```python
from build123d import *

# Parameters (mm, degrees)
CROQUIS1_W              = 365
CROQUIS1_H              = 80
SALIENTE_EXTRUIR1_DEPTH = 50
REDONDEO1_R             = 20
REDONDEO2_R             = 20
REDONDEO3_R             = 20
REDONDEO4_R             = 20
CROQUIS2_W              = 25
CROQUIS2_H              = 25
SALIENTE_EXTRUIR2_DEPTH = 27
CROQUIS3_W              = 19
CROQUIS3_H              = 19
CORTAR_EXTRUIR1_DEPTH   = 23


with BuildPart() as part:
    # Croquis1 → Saliente-Extruir1 (new body)
    with BuildSketch(Plane(origin=(0, 0, 0), x_dir=(1, 0, 0), z_dir=(0, 1, 0))):
        with Locations((-182.5, 40)):
            Rectangle(CROQUIS1_W, CROQUIS1_H)
    extrude(amount=SALIENTE_EXTRUIR1_DEPTH)

    # Redondeo1
    redondeo1_edges = [part.edges().sort_by_distance(p)[0] for p in [
        (-182.5, 50, -80),
    ]]
    fillet(redondeo1_edges, radius=REDONDEO1_R)

    # Redondeo2
    redondeo2_edges = [part.edges().sort_by_distance(p)[0] for p in [
        (-182.5, 50, 0),
    ]]
    fillet(redondeo2_edges, radius=REDONDEO2_R)

    # Redondeo3
    redondeo3_edges = [part.edges().sort_by_distance(p)[0] for p in [
        (0, 15, -80),
        (0, 44.142135624, -74.142135624),
        (0, 15, 0),
        (0, 50, -40),
        (0, 44.142135624, -5.857864376),
    ]]
    fillet(redondeo3_edges, radius=REDONDEO3_R)

    # Redondeo4
    redondeo4_edges = [part.edges().sort_by_distance(p)[0] for p in [
        (-365, 15, -80),
        (-365, 44.142135624, -74.142135624),
        (-365, 15, 0),
        (-365, 50, -40),
        (-365, 44.142135624, -5.857864376),
    ]]
    fillet(redondeo4_edges, radius=REDONDEO4_R)

    # Croquis2 → Saliente-Extruir2 (add)
    with BuildSketch(Plane.XZ):
        with Locations((-53.967193185, -38.316617584)):
            Rectangle(CROQUIS2_W, CROQUIS2_H)
    extrude(amount=SALIENTE_EXTRUIR2_DEPTH)

    # Croquis3 → Cortar-Extruir1 (cut)
    with BuildSketch(Plane.XZ.offset(27)):
        with Locations((-54, -38)):
            Rectangle(CROQUIS3_W, CROQUIS3_H)
    extrude(amount=-CORTAR_EXTRUIR1_DEPTH, mode=Mode.SUBTRACT)


solid = part.part
```
Design review of the part built by this model. Coordinates are the model's own, in mm. A direction names the side the tool comes from. Round coordinates to 2 decimals unless told otherwise and drop trailing zeros. Order: outer loops, then holes, each group sorted by start corner. A loop starts at its lowest first (then second) coordinate and runs counter-clockwise, first axis right, second up. Notation, with made-up numbers: (81.25, -21) - (124.25, -21) arc R24 cw to (124.25, 10) - close; hole circle Ø4 at (69, 62.25). An arc over 180 degrees is marked (long way). Return JSON: item names as keys, results as strings.
Q1. Machinability: for faces 1 (the flat face through (-66.467, -13, -38)), 2 (the flat face through (-54, -13, -50.817)), 3 (the flat face through (-54, -16, -47.5)), which of the approach directions +Z, -Z, +X, -X, +Y, -Y give a long, thin tool a straight path to every point of the face, cutting with its end or side? Answer none if there is none.
Computed values:
{"face 1": "+Z, -Z, -X, -Y", "face 2": "-Z, +X, -X, -Y", "face 3": "-Y"}
Q2. Wall thickness on L1, parallel to X at y = -21, z = -45; L2, parallel to Y at x = -161.5, z = -25.5; L3, parallel to X at y = 31, z = -21.5: over which ranges is each line inside the solid? List them lowest first. Write a range as [from, to].
Computed values:
{"L1": "x = [-66.47, -63.5], [-44.5, -41.47]", "L2": "y = [0, 50]", "L3": "x = [-364.97, -0.03]"}
Q3. Consider section C-C on z = -41. Write out the cut boundary in (x, y), plus the area to 3 significant figures.
Computed values:
{"outline": "(-365, 0) - (-66.47, 0) - (-66.47, -27) - (-63.5, -27) - (-63.5, -4) - (-44.5, -4) - (-44.5, -27) - (-41.47, -27) - (-41.47, 0) - (0, 0) - (0, 30) arc R20 ccw to (-20, 50) - (-345, 50) arc R20 ccw to (-365, 30) - close", "area": "18,300 mm2"}
Q4. Consider section B-B on x = -250.5. Write out the cut boundary in (y, z), plus the area to 3 significant figures.
Computed values:
{"outline": "(0, -80) - (30, -80) arc R20 ccw to (50, -60) - (50, -20) arc R20 ccw to (30, 0) - (0, 0) - close", "area": "3,830 mm2"}
Q5. Consider section A-A on y = -21.5. Write out the cut boundary in (x, z), plus the area to 3 significant figures.
Computed values:
{"outline": "(-66.47, -50.82) - (-41.47, -50.82) - (-41.47, -25.82) - (-66.47, -25.82) - close; hole (-63.5, -47.5) - (-44.5, -47.5) - (-44.5, -28.5) - (-63.5, -28.5) - close", "area": "264 mm2"}
Q6. Consider section D-D on y = 39.5. Write out the cut boundary in (x, z), plus the area to 3 significant figures.
Computed values:
{"outline": "(-362.6, -60) arc R17.6 ccw to (-345, -77.6) - (-20, -77.6) arc R17.6 ccw to (-2.4, -60) - (-2.4, -20) arc R17.6 ccw to (-20, -2.4) - (-345, -2.4) arc R17.6 ccw to (-362.6, -20) - close", "area": "26,800 mm2"}
Q7. For pin 1 Ø15 at (y, z) = (-13, -35) entering from -X; pin 2 Ø5.5 at (x, y) = (-54, -16.5) entering from +Z; pin 3 Ø12.5 at (x, y) = (-57.5, -13.5) entering from -Z, all flat-tipped, find the tip position at first contact; note any pin that passes through.
Computed values:
{"pin 1": "stops at x = -66.47", "pin 2": "stops at z = -25.82", "pin 3": "stops at z = -50.82"}
Q8. The part is to be moulded in two halves that separate along Z. For faces 4 (the flat face through (-54, -16, -28.5)), 5 (the flat face through (-65, -27, -38)), 6 (the cylindrical face through (-359.297, 15.21, -73.986)), say which applies: pulls with the +Z half, pulls with the -Z half, needs draft (parallel to the pull), parting line crosses it, or undercut.
Computed values:
{"face 4": "undercut", "face 5": "needs draft", "face 6": "pulls with the -Z half"}
